from build123d import *

# Parameters (mm, degrees)
SKETCH1_R           = 3
BOSS_EXTRUDE1_DEPTH = 3
SKETCH2_R           = 1.5
BOSS_EXTRUDE2_DEPTH = 4.3
FILLET1_R           = 0.5
SKETCH3_W           = 0.8
SKETCH3_H           = 1.1
SKETCH3_W_2         = 1.1
SKETCH3_H_2         = 0.8
CUT_EXTRUDE1_DEPTH  = 1


with BuildPart() as part:
    # Sketch1 → Boss-Extrude1 (new body)
    with BuildSketch(Plane(origin=(0, 0, 0), x_dir=(1, 0, 0), z_dir=(0, 1, 0))):
        with Locations(Location((0, 0, 0), (0, 0, 270))):
            Circle(SKETCH1_R)
    extrude(amount=BOSS_EXTRUDE1_DEPTH)

    # Sketch2 → Boss-Extrude2 (add)
    with BuildSketch(Plane.XZ):
        with Locations(Location((0, 0, 0), (0, 0, 90))):
            Circle(SKETCH2_R)
    extrude(amount=BOSS_EXTRUDE2_DEPTH)

    # Fillet1
    fillet1_edges = [part.edges().sort_by_distance(p)[0] for p in [
        (0, 3, -3),
    ]]
    fillet(fillet1_edges, radius=FILLET1_R)

    # Sketch3 → Cut-Extrude1 (cut)
    with BuildSketch(Plane(origin=(0, 3, 0), x_dir=(1, 0, 0), z_dir=(0, 1, 0))):
        with Locations((0, 0.95)):
            Rectangle(SKETCH3_W, SKETCH3_H)
        with Locations((0.95, 0)):
            Rectangle(SKETCH3_W_2, SKETCH3_H_2)
        with Locations((0, -0.95)):
            Rectangle(SKETCH3_W, SKETCH3_H)
        with Locations((-0.95, 0)):
            Rectangle(SKETCH3_W_2, SKETCH3_H_2)
        Rectangle(SKETCH3_W, SKETCH3_H_2)
    extrude(amount=-CUT_EXTRUDE1_DEPTH, mode=Mode.SUBTRACT)


solid = part.part
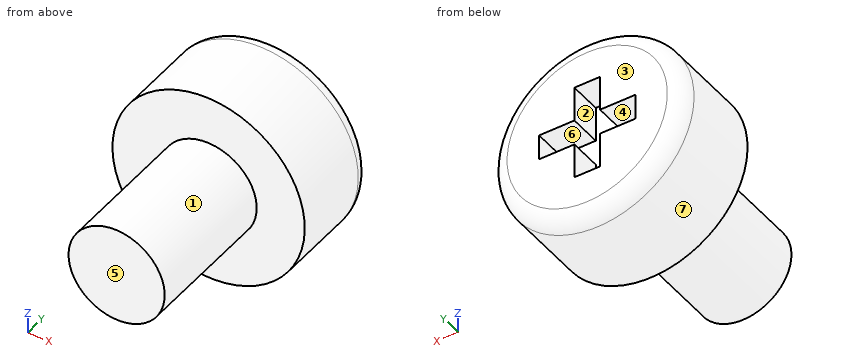
For this review, take the finished solid that the model builds, in its own axes (mm). Face numbers are marked on the shaded views. A direction names the side the tool comes from. Round coordinates to 2 decimals unless told otherwise and drop trailing zeros. Loops run counter-clockwise (first coordinate to the right, second up) from the corner with the lowest first, then second, coordinate; pieces in that order, holes last. Notation, with made-up numbers: (-13, -8.75) - (27, -8.75) arc R24 cw to (27, 30.25) - close; hole circle Ø10 at (50, -35.75). An arc over 180 degrees is marked (long way). Use one line per item in the form item = value.
1) Tool access review of the marked faces 1, 2 and 3: name each direction out of +Z, -Z, +X, -X, +Y, -Y from which nothing blocks a thin tool from reaching the whole face with its end or side.
Solutions:
face_1 = -Y
face_2 = +Y
face_3 = +Z, -Z, +X, -X, +Y
2) Wall thickness on probe 1 along X at (y, z) = (2.25, -0.1); probe 2 along Y at (x, z) = (0.8, 2.25); probe 3 along X at (y, z) = (2.75, -1.3): over which ranges is each line inside the solid? List them lowest first.
Solutions:
probe_1 = -3 to -1.5, 1.5 to 3
probe_2 = 0 to 3
probe_3 = -2.63 to -0.4, 0.4 to 2.63
3) Clearance check with flat-ended pins moving along their axes: P1, Ø1, axis at x = 1, y = 1, coming from the +Z side; P2, Ø3, axis at x = 1.5, y = -3.5, coming from the +Z side; P3, Ø0.8, axis at y = 2.5, z = -1, coming from the -X side. State where each tip first meets the part, or that it passes through.
Solutions:
P1 = 2.96
P2 = 1.5
P3 = -2.94
4) We need section B-B on y = 2.75. Write out the cut boundary in (x, z), then the cut area to 3 significant figures.
Solutions:
outline = circle Ø5.87 at (0, 0); hole (-1.5, -0.4) - (-0.4, -0.4) - (-0.4, -1.5) - (0.4, -1.5) - (0.4, -0.4) - (1.5, -0.4) - (1.5, 0.4) - (0.4, 0.4) - (0.4, 1.5) - (-0.4, 1.5) - (-0.4, 0.4) - (-1.5, 0.4) - close
area = 22.9 mm2
5) We need section C-C on z = 0. Write out the cut boundary in (x, y).
Solutions:
outline = (-3, 0) - (-1.5, 0) - (-1.5, -4.3) - (1.5, -4.3) - (1.5, 0) - (3, 0) - (3, 2.5) arc R0.5 ccw to (2.5, 3) - (1.5, 3) - (1.5, 2) - (-1.5, 2) - (-1.5, 3) - (-2.5, 3) arc R0.5 ccw to (-3, 2.5) - close
6) We need section D-D on y = -2.25. Write out the cut boundary in (x, z).
Solutions:
outline = circle Ø3 at (0, 0)
7) We need section A-A on x = 0. Write out the cut boundary in (y, z), then the cut area to 3 significant figures.
Solutions:
outline = (-4.3, -1.5) - (0, -1.5) - (0, -3) - (2.5, -3) arc R0.5 ccw to (3, -2.5) - (3, -1.5) - (2, -1.5) - (2, 1.5) - (3, 1.5) - (3, 2.5) arc R0.5 ccw to (2.5, 3) - (0, 3) - (0, 1.5) - (-4.3, 1.5) - close
area = 27.8 mm2
8) Mouldability with a two-part tool opening along X and no side actions: class the marked faces 4, 5, 6 and 7 as pulls with the +X half, pulls with the -X half, needs draft (parallel to the pull), parting line crosses it, or undercut.
Solutions:
face_4 = undercut
face_5 = needs draft
face_6 = undercut
face_7 = parting line crosses it
